The drawing under review shows one solid part. Ordinate dimensions are in mm from its lowest x, y, z. A direction names the side the tool comes from. Coordinates: 2 decimals unless noted, no trailing zeros. Order: outer loops, then holes, each group sorted by start corner. A loop starts at its lowest first (then second) coordinate and runs counter-clockwise, first axis right, second up.
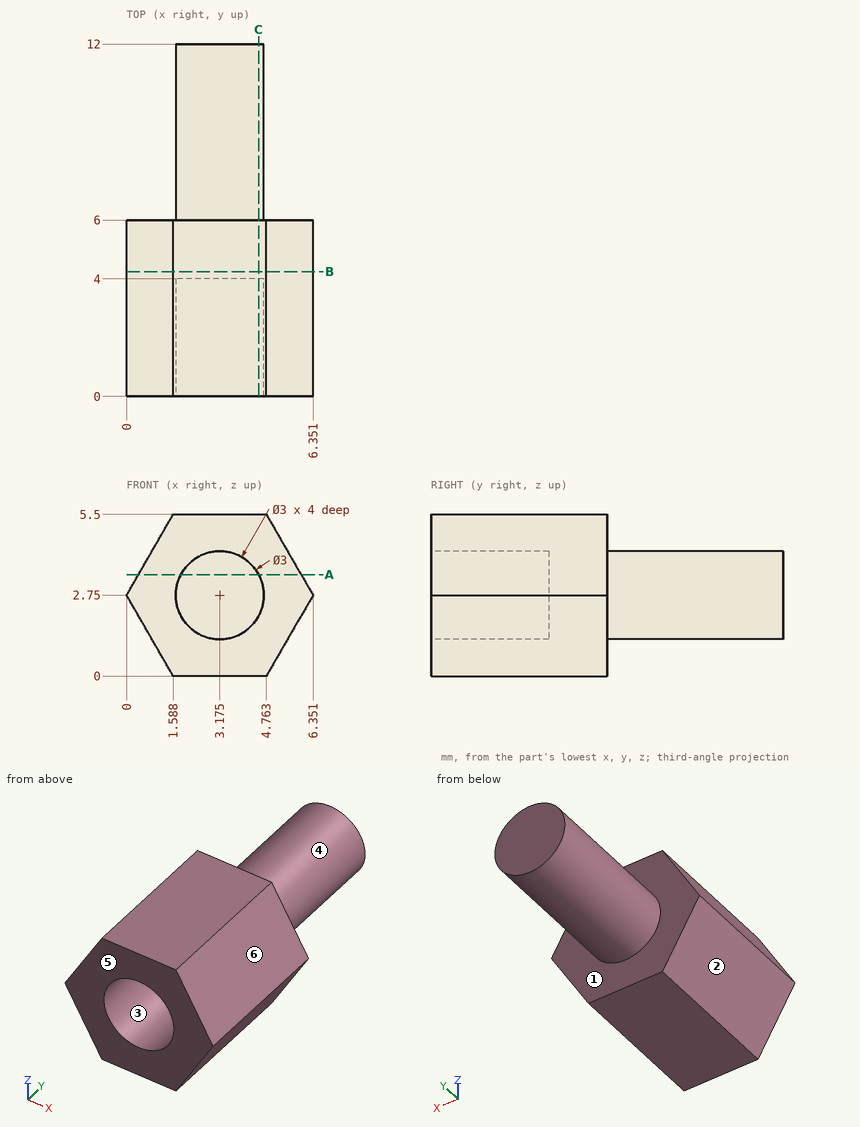
(1) Insertion check: pin 1 Ø1 at (y, z) = (8.5, 4) entering from -X; pin 2 Ø3 at (y, z) = (9, 1.5) entering from -X (1 decimal). Each pin has a flat end and moves straight along its axis. Give the tip position at first contact, or say it passes through.
(2) The part is to be moulded in two halves that separate along Z. For the marked faces 3, 4, 5 and 6, say which applies: +Z half, -Z half, draft (parallel to the pull), parting line (faces both ways), or undercut.
(3) Consider section B-B (y = 4.25). Give the boundary of the cut face in (x, z), then the cut area to 3 significant figures.
(4) Tool access review of the marked faces 1 and 2: name each direction out of +Z, -Z, +X, -X, +Y, -Y from which nothing blocks a thin tool from reaching the whole face with its end or side.
(5) Consider section C-C (x = 4.5). Give the boundary of the cut face in (y, z).
(6) Wall thickness on line 1 (Y direction, x = 3, z = 0.4); line 2 (Y direction, x = 3.25, z = 3.6); line 3 (Z direction, x = 4, y = 3.5) (1 decimal): over which ranges is each line inside the solid? List them lowest first.
(7) Consider section A-A (z = 3.45). Give the boundary of the cut face in (x, y) (1 decimal).
Findings:
1. pin 1: stops at x = 1.88
1. pin 2: stops at x = 1.7
2. face 3: undercut
2. face 4: parting line
2. face 5: draft
2. face 6: +Z half
3. outline: (0, 2.75) - (1.59, 0) - (4.76, 0) - (6.35, 2.75) - (4.76, 5.5) - (1.59, 5.5) - close
3. area: 26.2 mm2
4. face 1: +Y
4. face 2: -Z, -X, +Y, -Y
5. outline: (0, 0) - (6, 0) - (6, 2.05) - (12, 2.05) - (12, 3.45) - (6, 3.45) - (6, 5.5) - (0, 5.5) - (0, 3.45) - (4, 3.45) - (4, 2.05) - (0, 2.05) - close
6. line 1: y = 0 to 6
6. line 2: y = 4 to 12
6. line 3: z = 0 to 1.5, 4 to 5.5
7. outline: (0.4, 0) - (1.8, 0) - (1.8, 4) - (4.5, 4) - (4.5, 0) - (5.9, 0) - (5.9, 6) - (4.5, 6) - (4.5, 12) - (1.8, 12) - (1.8, 6) - (0.4, 6) - close
